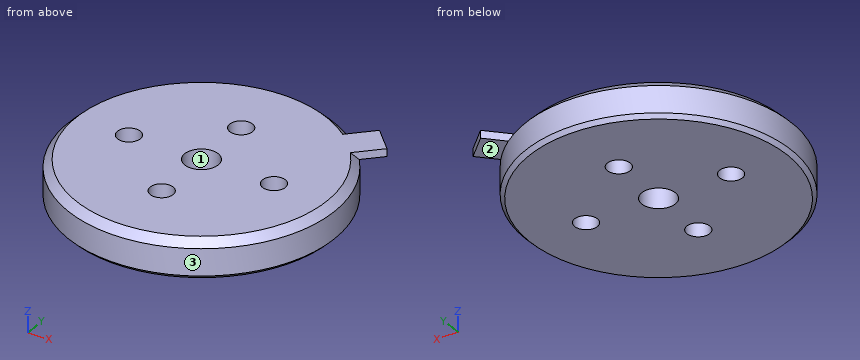
```python
from build123d import *

# Parameters (mm, degrees)
F0_R     = 17.4
F0_R_2   = 1.5
F0_R_3   = 2.2
F1_DEPTH = 5
F2_SIZE  = 1
F3_SIZE  = 0.5
F5_DEPTH = 1


with BuildPart() as f1:
    # F0 (on Top) → F1 (new body)
    with BuildSketch(Plane.XY):
        Circle(F0_R)
        with Locations((0, -8)):
            Circle(F0_R_2, mode=Mode.SUBTRACT)
        with Locations((-9.5, 0)):
            Circle(F0_R_2, mode=Mode.SUBTRACT)
        Circle(F0_R_3, mode=Mode.SUBTRACT)
        with Locations((0, 8)):
            Circle(F0_R_2, mode=Mode.SUBTRACT)
        with Locations((9.5, 0)):
            Circle(F0_R_2, mode=Mode.SUBTRACT)
    extrude(amount=F1_DEPTH)

    # F2
    f2_edges = [f1.edges().sort_by_distance(p)[0] for p in [
        (-17.4, 0, 5),
    ]]
    chamfer(f2_edges, length=F2_SIZE)

    # F3
    f3_edges = [f1.edges().sort_by_distance(p)[0] for p in [
        (-17.4, 0, 0),
    ]]
    chamfer(f3_edges, length=F3_SIZE)

    # F4 (on face) → F5 (join)
    with BuildSketch(Plane.XY.offset(5)):
        Polygon((13.010765, 15.839192), (9.828784, 12.657211), (12.657211, 9.828784), (15.839192, 13.010765), align=None)
    extrude(amount=-F5_DEPTH)


solid = f1.part
```
Check sheet for the modelled part. Datum: model origin and axes. Units: mm. Face numbers are marked on the shaded views. Coordinates: 2 decimals unless noted, no trailing zeros. Loops run counter-clockwise (first coordinate to the right, second up) from the corner with the lowest first, then second, coordinate; pieces in that order, holes last. Notation, with made-up numbers: M 28.25,-37 L 74.25,-37 A15 ccw 74.25,-22 Z; hole C 61,31.5 d10. An arc over 180 degrees is marked long. Answer as a JSON object with one key per item and string values.
1. Sectioned sample at B-B on x = 0. Record the cut outline in (y, z), and give its area (3 significant figures).
Outcome:
{"outline": "M -17.4,0.5 L -16.9,0 L -9.5,0 L -9.5,5 L -16.4,5 L -17.4,4 Z; M -6.5,0 L -2.2,0 L -2.2,5 L -6.5,5 Z; M 2.2,0 L 6.5,0 L 6.5,5 L 2.2,5 Z; M 9.5,0 L 16.9,0 L 17.4,0.5 L 17.4,4 L 16.4,5 L 9.5,5 Z", "area": "121 mm²"}
2. Scan lines: L1, parallel to Y at x = 0, z = 3.3; L2, parallel to Y at x = -0.5, z = 4.6; L3, parallel to Y at x = -9, z = 2.9. Record each from-to range of solid material in increasing order. Write a range as from..to.
Outcome:
{"L1": "-17.4..-9.5, -6.5..-2.2, 2.2..6.5, 9.5..17.4", "L2": "-16.79..-9.41, -6.59..-2.14, 2.14..6.59, 9.41..16.79", "L3": "-14.89..-1.41, 1.41..14.89"}
3. Release check for a two-part mould opening along Y. For the marked faces 1, 2 and 3 record: pulls with the +Y half, pulls with the -Y half, needs draft (parallel to the pull), parting line crosses it, or undercut.
Outcome:
{"face 1": "undercut", "face 2": "needs draft", "face 3": "parting line crosses it"}
4. Sectioned sample at C-C on z = 3.6. Record the cut outline in (x, y).
Outcome:
{"outline": "C 0,0 d34.8; hole C -9.5,0 d3; hole C 0,0 d4.4; hole C 0,-8 d3; hole C 0,8 d3; hole C 9.5,0 d3"}
5. Sectioned sample at A-A on y = 0. Record the cut outline in (x, z).
Outcome:
{"outline": "M -17.4,0.5 L -16.9,0 L -11,0 L -11,5 L -16.4,5 L -17.4,4 Z; M -8,0 L -2.2,0 L -2.2,5 L -8,5 Z; M 2.2,0 L 8,0 L 8,5 L 2.2,5 Z; M 11,0 L 16.9,0 L 17.4,0.5 L 17.4,4 L 16.4,5 L 11,5 Z"}
6. Depth check by flat-ended pin: P1, Ø1, axis at x = -11, z = 3.5, coming from the +Y side; P2, Ø1.5, axis at x = 13.5, y = 14, coming from the -Z side; P3, Ø2, axis at x = -9, z = 1, coming from the +Y side. Enter the tip coordinate at first touch or a pass-through.
Outcome:
{"P1": "y = 13.87", "P2": "z = 4", "P3": "y = 15.45"}
